Here's the drawing with two shaded views (mm, measured from the low corner). I have some questions. A direction names the side the tool comes from. Round coordinates to 2 decimals unless told otherwise and drop trailing zeros. Write each loop counter-clockwise with the first axis right and the second up, starting at its lowest first coordinate (ties: lowest second). Pieces come first, ordered by that corner, then holes. Notation, with made-up numbers: M -32.5,84.5 L -15.5,84.5 A12 cw -15.5,107.5 Z; hole C 1,19.5 d5. An arc over 180 degrees is marked long. Write item = value, one per line. Start each with the question number.
(1) On a 3-axis mill with a long thin cutter (end or side, diameter ignored), from which of +Z, -Z, +X, -X, +Y, -Y can I reach the whole of each face in a straight line? I mean the marked faces 4 and 5. Say none if no direction works.
(2) I want a section at C-C (x = 3.55). List the corners of the cut face in (y, z) for me (1 decimal).
(3) I want a section at B-B (y = 12). List the corners of the cut face in (x, z) for me (1 decimal).
(4) I want a section at D-D (z = 0.5). List the corners of the cut face in (x, y) for me, and give its area (3 significant figures).
(5) I need wall thicknesses on line 1 along Y through (x, z) = (0.2, 1.75); line 2 along Y through (x, z) = (2.8, 3.8); line 3 along X through (y, z) = (7.75, 2.2). Which ranges of each line are inside material? Lowest first, please.
(6) I want a section at A-A (y = 6.5). List the corners of the cut face in (x, z) for me.
(7) If we mould it in two halves opening along X, with no side actions, what happens to the marked faces 1, 2 and 3? For each: released by +X, released by -X, zero draft, split by the parting line, or undercut.
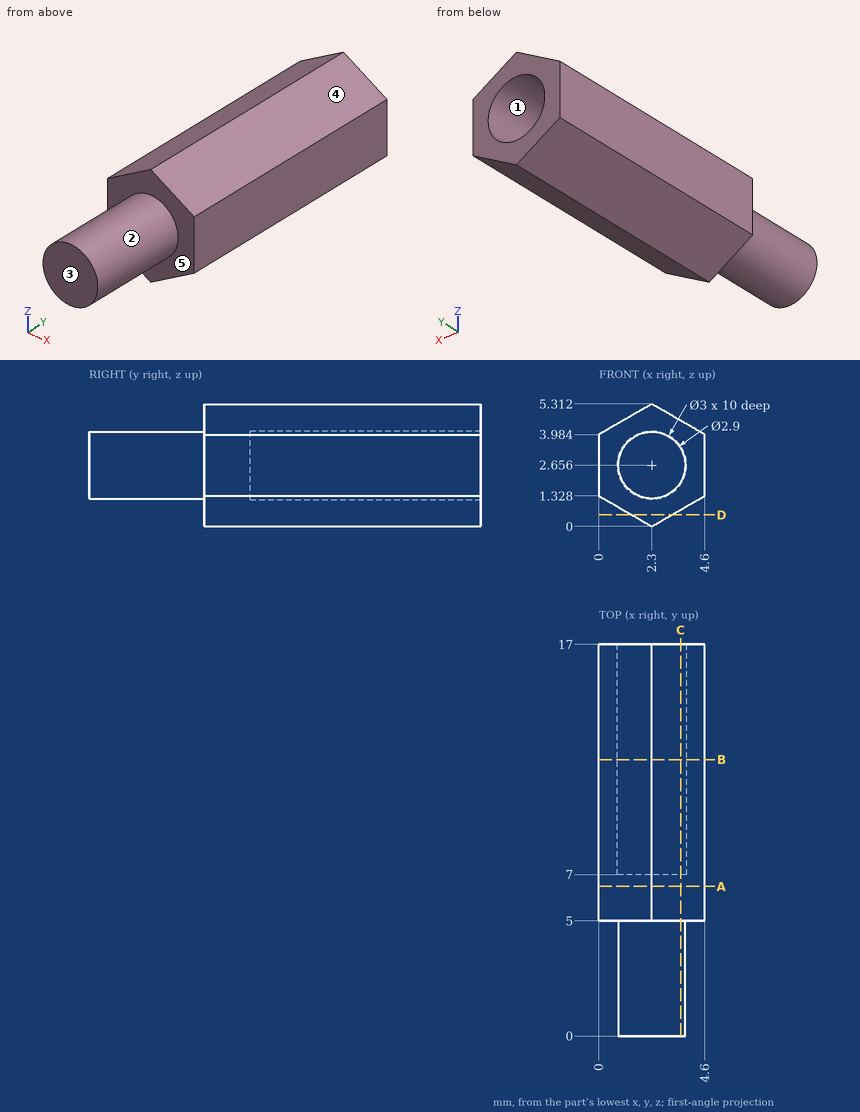
Returned:
q1.face_4 = +Z, +X, +Y, -Y
q1.face_5 = -Y
q2.outline = M 0,1.9 L 5,1.9 L 5,0.7 L 17,0.7 L 17,1.8 L 7,1.8 L 7,3.5 L 17,3.5 L 17,4.6 L 5,4.6 L 5,3.4 L 0,3.4 Z
q3.outline = M 0,1.3 L 2.3,0 L 4.6,1.3 L 4.6,4 L 2.3,5.3 L 0,4 Z; hole C 2.3,2.7 d3
q4.outline = M 1.43,5 L 3.17,5 L 3.17,17 L 1.43,17 Z
q4.area = 20.8 mm²
q5.line_1 = 5 to 17
q5.line_2 = 0 to 7
q5.line_3 = 0 to 0.87, 3.73 to 4.6
q6.outline = M 0,1.33 L 2.3,0 L 4.6,1.33 L 4.6,3.98 L 2.3,5.31 L 0,3.98 Z
q7.face_1 = undercut
q7.face_2 = split by the parting line
q7.face_3 = zero draft
